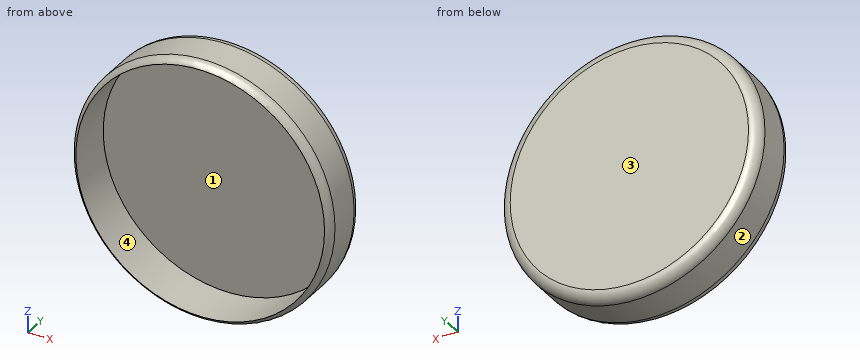
from build123d import *

# Parameters (mm, degrees)
F0_R     = 63.5
F1_DEPTH = 25.4
F2_T     = -2.54


# Not quite as in the source:
# - a fillet or chamfer that OpenCascade refuses, or shapes differently, is made with other operations: its cross-section is extruded or revolved along the edge and cut away or added


with BuildPart() as f1:
    # F0 (on Front) → F1 (new body)
    with BuildSketch(Plane.XZ):
        Circle(F0_R)
    extrude(amount=F1_DEPTH)

    # F2
    f2_openings = [f1.faces().sort_by_distance(p)[0] for p in [
        (0, -25.4, 0),
    ]]
    offset(amount=F2_T, openings=f2_openings)

    # F3: fillet of radius 5.08 on 3 edges, made by hand

    # F3_s1 → F3_t2 (revolve, cut)
    with BuildSketch(Plane.XY):
        with BuildLine():
            ThreePointArc((63.5, -5.08), (62.0121024484, -1.4878975516), (58.42, 0))
            Line((58.42, 0), (63.5, 0))
            Line((63.5, 0), (63.5, -5.08))
        make_face()
    revolve(axis=Axis((0, 0, 0), (0, -1, 0)), mode=Mode.SUBTRACT)

    # F3_s3 → F3_t4 (revolve, cut)
    with BuildSketch(Plane.XY):
        with BuildLine():
            ThreePointArc((63.5, -21.0005909488), (62.8194090512, -23.5405909488), (60.96, -25.4))
            Line((60.96, -25.4), (63.5, -25.4))
            Line((63.5, -25.4), (63.5, -21.0005909488))
        make_face()
    revolve(axis=Axis((0, -25.4, 0), (0, -1, 0)), mode=Mode.SUBTRACT)


solid = f1.part
Model file for the job. Use its own axes, mm. Face numbers are marked on the shaded views. Coordinates: 2 decimals unless noted, no trailing zeros. Write each loop counter-clockwise with the first axis right and the second up, starting at its lowest first coordinate (ties: lowest second). Pieces come first, ordered by that corner, then holes. Notation, with made-up numbers: (52, -12.5) -> (83, -12.5) arc R7 ccw to (83, -8.5) -> close; hole circle Ø4 at (82, -13). An arc over 180 degrees is marked (long way). One line per item, written item: value. Start each with the question number.
1) Probe probe 1 along Z at (x, y) = (0, -14); probe 2 along X at (y, z) = (-4.25, 17.5); probe 3 along Z at (x, y) = (-20.5, -7). List the from-to ranges inside material, lowest first.
2) Slice it at A-A on x = 0. Write the cut outline in (y, z), then the cut area to 3 significant figures.
3) Flat gauge pins, fed straight in: pin 1 Ø8 at (x, y) = (-42, -17) entering from +Z; pin 2 Ø10 at (x, y) = (43.5, -14.5) entering from -Z; pin 3 Ø1 at (y, z) = (-12.5, 8.5) entering from -X. Where does each tip first touch, or does it go through?
4) Pull direction Z, two halves, no side cores. Call the marked faces 1, 2, 3 and 4: +Z half, -Z half, draft (parallel to the pull), parting line (faces both ways), or undercut.
5) Slice it at C-C on y = -9. Write the cut outline in (x, z), then the cut area to 3 significant figures.
6) Slice it at B-B on z = 0. Write the cut outline in (x, y), then the cut area to 3 significant figures.
Answers follow:
1. probe 1: -63.5 to -60.96, 60.96 to 63.5
1. probe 2: -60.97 to -58.39, 58.39 to 60.97
1. probe 3: -60.1 to -57.41, 57.41 to 60.1
2. outline: (-25.4, -60.96) arc R5.08 ccw to (-21, -63.5) -> (-5.08, -63.5) arc R5.08 ccw to (0, -58.42) -> (0, 58.42) arc R5.08 ccw to (-5.08, 63.5) -> (-21, 63.5) arc R5.08 ccw to (-25.4, 60.96) -> (-2.54, 60.96) -> (-2.54, -60.96) -> close
2. area: 421 mm2
3. pin 1: z = 50.87
3. pin 2: z = -50.5
3. pin 3: x = -62.99
4. face 1: undercut
4. face 2: parting line
4. face 3: draft
4. face 4: undercut
5. outline: circle Ø127 at (0, 0); hole circle Ø121.92 at (0, 0)
5. area: 993 mm2
6. outline: (-63.5, -21) arc R5.08 ccw to (-60.96, -25.4) -> (-60.96, -2.54) -> (60.96, -2.54) -> (60.96, -25.4) arc R5.08 ccw to (63.5, -21) -> (63.5, -5.08) arc R5.08 ccw to (58.42, 0) -> (-58.42, 0) arc R5.08 ccw to (-63.5, -5.08) -> close
6. area: 421 mm2
